Here's how the part is built. I have some questions about the finished solid (model axes, mm). Face numbers are marked on the shaded views. A direction names the side the tool comes from. Give positions to 0.01 mm unless a question says otherwise; leave off trailing zeros. Loops run counter-clockwise (first coordinate to the right, second up) from the corner with the lowest first, then second, coordinate; pieces in that order, holes last. Notation, with made-up numbers: M -36,33 L 11,33 A22 ccw 11,68 Z; hole C 86.5,70.25 d4. An arc over 180 degrees is marked long. Answer as CSV lines item,"result". Start each with the question number.
Item 1: I want a section at C-C on z = -10.16. List the corners of the cut face in (x, y) for me (3 decimals).
Item 2: For the marked faces 1 and 2, which set-ups out of +Z, -Z, +X, -X, +Y, -Y let a thin tool reach every point of the face, with its end or its side?
Item 3: If I drill on line 1 along Z through (x, y) = (-8.89, -23.45); line 2 along Z through (x, y) = (-8, -24); line 3 along Z through (x, y) = (-7.5, 18) (3 decimals), over which ranges is the centre line in solid material (lowest first)? Write a range as from..to.
Item 4: Will these pins go through, and if not, where does the flat tip stop? P1, Ø6.5, axis at x = 8.89, z = -27.94, coming from the +Y side (3 decimals); P2, Ø3, axis at x = 11.5, y = 6.5, coming from the -Z side; P3, Ø3, axis at y = -19.5, z = -13, coming from the -X side; P4, Ø5, axis at x = 13, z = -3.5, coming from the +Y side.
Item 5: I want a section at D-D on x = 8.89. List the corners of the cut face in (y, z) for me (3 decimals), plus the area to 3 significant figures.
Item 6: I want a section at B-B on x = 0. List the corners of the cut face in (y, z) for me (1 decimal), plus the area to 3 significant figures.
from build123d import *

# Parameters (mm, degrees)
SKETCH1_W              = 38.1
SKETCH1_H              = 50.8
SKETCH1_R              = 14.2875
BOSS_EXTRUDE1_DEPTH    = 3.175
SKETCH2_W              = 38.1
SKETCH2_H              = 3.175
BOSS_EXTRUDE2_DEPTH    = 38.1
SKETCH3_R              = 2.413
CUT_EXTRUDE1_DEPTH     = 64.895642457
CONVERT_SOLID1_START   = -19.05
CONVERT_SOLID1_DEPTH   = 38.1
CONVERT_SOLID1_2_DEPTH = 38.1
FILLET1_R              = 2.54


# Read off the part's stored shape, not the designer's step: Convert-Solid1
with BuildPart() as part:
    # Sketch1 → Boss-Extrude1 (new body)
    with BuildSketch(Plane.XY):
        Rectangle(SKETCH1_W, SKETCH1_H)
        Circle(SKETCH1_R, mode=Mode.SUBTRACT)
    extrude(amount=BOSS_EXTRUDE1_DEPTH)

    # Sketch2 → Boss-Extrude2 (add)
    with BuildSketch(Plane(origin=(0, 0, 0), x_dir=(-1, 0, 0), z_dir=(0, 0, -1))):
        with Locations((0, -23.8125)):
            Rectangle(SKETCH2_W, SKETCH2_H)
    extrude(amount=BOSS_EXTRUDE2_DEPTH)

    # Sketch3 → Cut-Extrude1 (cut, through all)
    with BuildSketch(Plane(origin=(0, -22.225, 0), x_dir=(1, 0, 0), z_dir=(0, 1, 0))):
        with Locations(Location((-8.89, 27.94, 0), (0, 0, 180))):
            Circle(SKETCH3_R)
        with Locations(Location((8.89, 27.94, 0), (0, 0, 180))):
            Circle(SKETCH3_R)
        with Locations(Location((-8.89, 10.16, 0), (0, 0, 180))):
            Circle(SKETCH3_R)
        with Locations(Location((8.89, 10.16, 0), (0, 0, 180))):
            Circle(SKETCH3_R)
    extrude(amount=-CUT_EXTRUDE1_DEPTH, mode=Mode.SUBTRACT)

    # Convert-Solid1 outline → Convert-Solid1 (cut)
    with BuildSketch(Plane.YZ.offset(CONVERT_SOLID1_START)):
        with BuildLine():
            ThreePointArc((-25.4, -2.380000066), (-23.77297815, 1.54797815), (-19.844999934, 3.175))
            Line((-19.844999934, 3.175), (-25.4, 3.175))
            Line((-25.4, 3.175), (-25.4, -2.380000066))
        make_face()
    extrude(amount=CONVERT_SOLID1_DEPTH, mode=Mode.SUBTRACT)

    # Convert-Solid1 2 outline → Convert-Solid1 2 (add)
    with BuildSketch(Plane.YZ.offset(CONVERT_SOLID1_START)):
        with BuildLine():
            ThreePointArc((-22.225, -2.380000066), (-21.52791412, -0.69708588), (-19.844999934, 0))
            Line((-19.844999934, 0), (-22.225, 0))
            Line((-22.225, 0), (-22.225, -2.380000066))
        make_face()
    extrude(amount=CONVERT_SOLID1_2_DEPTH)

    # Fillet1
    fillet1_edges = [part.edges().sort_by_distance(p)[0] for p in [
        (19.05, 25.4, 1.5875),
        (-19.05, 25.4, 1.5875),
        (-19.05, -23.8125, -38.1),
        (19.05, -23.8125, -38.1),
    ]]
    fillet(fillet1_edges, radius=FILLET1_R)


solid = part.part
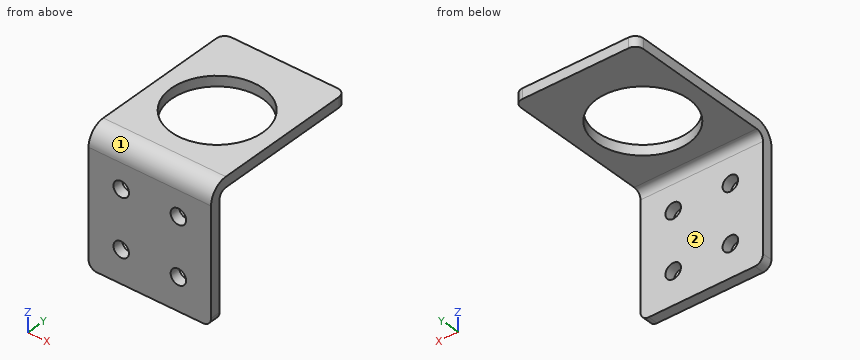
Result:
1,outline,"M -19.05,-25.4 L -11.303,-25.4 L -11.303,-22.225 L -19.05,-22.225 Z; M -6.477,-25.4 L 6.477,-25.4 L 6.477,-22.225 L -6.477,-22.225 Z; M 11.303,-25.4 L 19.05,-25.4 L 19.05,-22.225 L 11.303,-22.225 Z"
2,face 1,"+Z, +X, -X, -Y"
2,face 2,"-Z, +X, -X, +Y"
3,line 1,"-38.1..-30.35, -25.53..-12.57, -7.75..1.85"
3,line 2,"-38.1..-30.18, -25.7..-12.4, -7.92..1.31"
3,line 3,"0..3.175"
4,P1,"y = -22.225"
4,P2,"z = 0"
4,P3,"through"
4,P4,"y = -21.78"
5,outline,"M -25.4,-38.1 L -22.225,-38.1 L -22.225,-30.353 L -25.4,-30.353 Z; M -25.4,-25.527 L -22.225,-25.527 L -22.225,-12.573 L -25.4,-12.573 Z; M -25.4,-7.747 L -22.225,-7.747 L -22.225,-2.38 A2.38 cw -19.845,0 L -11.185,0 L -11.185,3.175 L -19.845,3.175 A5.555 ccw -25.4,-2.38 Z; M 11.185,0 L 25.4,0 L 25.4,3.175 L 11.185,3.175 Z"
5,area,"175 mm^2"
6,outline,"M -25.4,-38.1 L -22.2,-38.1 L -22.2,-2.4 A2.4 cw -19.8,0 L -14.3,0 L -14.3,3.2 L -19.8,3.2 A5.6 ccw -25.4,-2.4 Z; M 14.3,0 L 25.4,0 L 25.4,3.2 L 14.3,3.2 Z"
6,area,"186 mm^2"
